Verification items for the finished model (mm, model axes). Give positions to 0.01 mm unless a question says otherwise; leave off trailing zeros. Write each loop counter-clockwise with the first axis right and the second up, starting at its lowest first coordinate (ties: lowest second). Pieces come first, ordered by that corner, then holes. Notation, with made-up numbers: M 49.5,-28 L 101.5,-28 A32 cw 101.5,0 Z; hole C 61.25,16 d10. An arc over 180 degrees is marked long. Answer as a JSON object with one key per item and string values.
```python
from build123d import *

# Parameters (mm, degrees)
SKETCH1_W           = 122
SKETCH1_H           = 31
BOSS_EXTRUDE1_DEPTH = 9.7
SKETCH3_W           = 52
SKETCH3_H           = 27
CUT_EXTRUDE2_DEPTH  = 6.7
SKETCH4_W           = 3
SKETCH4_H           = 3
BOSS_EXTRUDE2_DEPTH = 2
CHAMFER1_SIZE       = 1
SKETCH5_R           = 1.75
CUT_EXTRUDE3_DEPTH  = 64.681551489


with BuildPart() as part:
    # Sketch1 → Boss-Extrude1 (new body)
    with BuildSketch(Plane(origin=(0, 0, 0), x_dir=(1, 0, 0), z_dir=(0, 1, 0))):
        Rectangle(SKETCH1_W, SKETCH1_H)
    extrude(amount=BOSS_EXTRUDE1_DEPTH)

    # Sketch3 → Cut-Extrude2 (cut)
    with BuildSketch(Plane(origin=(0, 9.7, 0), x_dir=(1, 0, 0), z_dir=(0, 1, 0))):
        with Locations((-28, 0)):
            Rectangle(SKETCH3_W, SKETCH3_H)
        with Locations((28, 0)):
            Rectangle(SKETCH3_W, SKETCH3_H)
    extrude(amount=-CUT_EXTRUDE2_DEPTH, mode=Mode.SUBTRACT)

    # Sketch4 → Boss-Extrude2 (add)
    with BuildSketch(Plane(origin=(0, 9.7, 0), x_dir=(1, 0, 0), z_dir=(0, 1, 0))):
        with Locations((-52.5, 14)):
            Rectangle(SKETCH4_W, SKETCH4_H)
        with Locations((-3.5, 14)):
            Rectangle(SKETCH4_W, SKETCH4_H)
        with Locations((-3.5, -14)):
            Rectangle(SKETCH4_W, SKETCH4_H)
        with Locations((-52.5, -14)):
            Rectangle(SKETCH4_W, SKETCH4_H)
        with Locations((52.5, -14)):
            Rectangle(SKETCH4_W, SKETCH4_H)
        with Locations((3.5, -14)):
            Rectangle(SKETCH4_W, SKETCH4_H)
        with Locations((3.5, 14)):
            Rectangle(SKETCH4_W, SKETCH4_H)
        with Locations((52.5, 14)):
            Rectangle(SKETCH4_W, SKETCH4_H)
    extrude(amount=-BOSS_EXTRUDE2_DEPTH)

    # Chamfer1
    chamfer1_edges = [part.edges().sort_by_distance(p)[0] for p in [
        (-52.5, 9.7, 12.5),
        (-3.5, 9.7, 12.5),
        (52.5, 9.7, 12.5),
        (3.5, 9.7, 12.5),
        (52.5, 9.7, -12.5),
        (3.5, 9.7, -12.5),
        (-3.5, 9.7, -12.5),
        (-52.5, 9.7, -12.5),
    ]]
    chamfer(chamfer1_edges, length=CHAMFER1_SIZE)

    # Sketch5 → Cut-Extrude3 (cut, through all)
    with BuildSketch(Plane(origin=(0, 9.7, 0), x_dir=(1, 0, 0), z_dir=(0, 1, 0))):
        with Locations(Location((-57.5, -10.5, 0), (0, 0, 270))):
            Circle(SKETCH5_R)
        with Locations(Location((57.5, 10.5, 0), (0, 0, 270))):
            Circle(SKETCH5_R)
    extrude(amount=-CUT_EXTRUDE3_DEPTH, mode=Mode.SUBTRACT)


solid = part.part
```
1) Release check for a two-part mould opening along Z. For faces 1 (the face through (61, 5, 0)), 2 (the face through (-1, 5, 15.5)), 3 (the face through (28, 3, 0)) record: pulls with the +Z half, pulls with the -Z half, needs draft (parallel to the pull), parting line crosses it, or undercut.
Completed:
{"face 1": "needs draft", "face 2": "pulls with the +Z half", "face 3": "undercut"}
2) Thickness scan on L1, parallel to X at y = 7.25, z = 10.5; L2, parallel to X at y = 6, z = -10.5; L3, parallel to X at y = 3.75, z = -5.5. Record the ranges inside material, lowest first.
Completed:
{"L1": "x = -61 to -59.25, -55.75 to -54, -2 to 2, 54 to 61", "L2": "x = -61 to -54, -2 to 2, 54 to 55.75, 59.25 to 61", "L3": "x = -61 to -54, -2 to 2, 54 to 61"}
3) Section check A-A on x = 57.5. Record the boundary of the cut face in (y, z).
Completed:
{"outline": "M 0,-15.5 L 9.7,-15.5 L 9.7,-12.25 L 0,-12.25 Z; M 0,-8.75 L 9.7,-8.75 L 9.7,15.5 L 0,15.5 Z"}
4) Go/stop test with a flat-tipped pin: pin 1 (3 mm diameter, centred on x = -40.5, z = 5.5, fed in from +Y). Record where the tip stops, or that it passes through.
Completed:
{"pin 1": "stops at y = 3"}
5) Section check C-C on z = -5. Record the boundary of the cut face in (x, y), and give its area (3 significant figures).
Completed:
{"outline": "M -61,0 L 61,0 L 61,9.7 L 54,9.7 L 54,3 L 2,3 L 2,9.7 L -2,9.7 L -2,3 L -54,3 L -54,9.7 L -61,9.7 Z", "area": "487 mm2"}
6) Section check D-D on x = -16. Record the boundary of the cut face in (y, z), and give its area (3 significant figures).
Completed:
{"outline": "M 0,-15.5 L 9.7,-15.5 L 9.7,-13.5 L 3,-13.5 L 3,13.5 L 9.7,13.5 L 9.7,15.5 L 0,15.5 Z", "area": "120 mm2"}
7) Section check B-B on z = -10.5. Record the boundary of the cut face in (x, y), and give its area (3 significant figures).
Completed:
{"outline": "M -61,0 L 55.75,0 L 55.75,9.7 L 54,9.7 L 54,3 L 2,3 L 2,9.7 L -2,9.7 L -2,3 L -54,3 L -54,9.7 L -61,9.7 Z; M 59.25,0 L 61,0 L 61,9.7 L 59.25,9.7 Z", "area": "453 mm2"}
